from build123d import *

# Parameters (mm, degrees)
BOSS_EXTRUDE1_DEPTH      = 20
BOSS_EXTRUDE1_DEPTH_BACK = 20
SKETCH1_R                = 8
BOSS_EXTRUDE2_DEPTH      = 20
BOSS_EXTRUDE2_DEPTH_BACK = 20
SKETCH3_R                = 8


with BuildPart() as part:
    # Sketch1 → Boss-Extrude1 (new, two sides: drawn at the far end of the back side and taken through both)
    with BuildSketch(Plane(origin=(0, 0, 0), x_dir=(1, 0, 0), z_dir=(0, 1, 0)).offset(-BOSS_EXTRUDE1_DEPTH_BACK)):
        with Locations(Location((0, 0, 0), (0, 0, 270))):
            Circle(SKETCH1_R)
    extrude(amount=BOSS_EXTRUDE1_DEPTH + BOSS_EXTRUDE1_DEPTH_BACK)

    # Sketch3 → Boss-Extrude2 (add, two sides: drawn at the far end of the back side and taken through both)
    with BuildSketch(Plane(origin=(0, 0, 0), x_dir=(0, 0, -1), z_dir=(1, 0, 0)).offset(-BOSS_EXTRUDE2_DEPTH_BACK)):
        Circle(SKETCH3_R)
    extrude(amount=BOSS_EXTRUDE2_DEPTH + BOSS_EXTRUDE2_DEPTH_BACK)


solid = part.part
Verification items for the finished model (mm, model axes). A direction names the side the tool comes from. Round coordinates to 2 decimals unless told otherwise and drop trailing zeros. Write each loop counter-clockwise with the first axis right and the second up, starting at its lowest first coordinate (ties: lowest second). Pieces come first, ordered by that corner, then holes.
(1) Section check C-C (x = 17). Enter the section's corners in (y, z), plus the area to 3 significant figures.
Returned:
outline: circle Ø16 at (0, 0)
area: 201 mm2
(2) Section check A-A (z = 0). Enter the section's corners in (x, y).
Returned:
outline: (-20, -8) - (-8, -8) - (-8, -20) - (8, -20) - (8, -8) - (20, -8) - (20, 8) - (8, 8) - (8, 20) - (-8, 20) - (-8, 8) - (-20, 8) - close
(3) Material ranges on line 1 (Y direction, x = -12, z = 0.25); line 2 (Z direction, x = -10, y = 3.5); line 3 (Y direction, x = -7, z = -6.5), recorded low to high.
Returned:
line 1: y = -8 to 8
line 2: z = -7.19 to 7.19
line 3: y = -4.66 to 4.66
(4) Section check B-B (y = 5). Enter the section's corners in (x, z) (3 decimals), plus the area to 3 significant figures.
Returned:
outline: (-20, -6.245) - (-5, -6.245) arc R8 ccw to (5, -6.245) - (20, -6.245) - (20, 6.245) - (5, 6.245) arc R8 ccw to (-5, 6.245) - (-20, 6.245) - close
area: 524 mm2
(5) Access from +Z, -Z, +X, -X, +Y, -Y to the whole of each face (thin tool, end or side, straight path). Record for faces 1 (the cylindrical face through (12, 0, 8)), 2 (the cylindrical face through (0, 12, -8)), 3 (the cylindrical face through (-4.868, -12.362, -6.349)), 4 (the flat face through (0, 20, 0)), 5 (the cylindrical face through (-12.362, -4.868, 6.349)).
Returned:
face 1: +X
face 2: +Y
face 3: -Y
face 4: +Z, -Z, +X, -X, +Y
face 5: -X
(6) Depth check by flat-ended pin: pin 1 Ø1.5 at (x, z) = (-7.5, -3.5) entering from -Y; pin 2 Ø1 at (x, y) = (5.5, 2.5) entering from -Z; pin 3 Ø5 at (y, z) = (-10, -4.5) entering from +X; pin 4 Ø2 at (y, z) = (-13.5, -2) entering from +X. Enter the tip coordinate at first touch or a pass-through.
Returned:
pin 1: stops at y = -20
pin 2: stops at z = -7.75
pin 3: stops at x = 7.75
pin 4: stops at x = 7.94
(7) Section check D-D (z = 4). Enter the section's corners in (x, y).
Returned:
outline: (-20, -6.93) - (-6.93, -6.93) - (-6.93, -20) - (6.93, -20) - (6.93, -6.93) - (20, -6.93) - (20, 6.93) - (6.93, 6.93) - (6.93, 20) - (-6.93, 20) - (-6.93, 6.93) - (-20, 6.93) - close
